Source: CAD feature listing. Evaluate the final solid. Frame: model axes, mm. A direction names the side the tool comes from. Give positions to 0.01 mm unless a question says otherwise; leave off trailing zeros.
from build123d import *

# Parameters (mm, degrees)
SKETCH1_R           = 2.4
BOSS_EXTRUDE1_DEPTH = 3.6


with BuildPart() as part:
    # Top → Base (revolve)
    with BuildSketch(Plane(origin=(0, 0, 0), x_dir=(1, 0, 0), z_dir=(0, 1, 0)), mode=Mode.PRIVATE) as base_sk:
        Polygon((-8.5, 32.9), (-8.5, 37.5), (-7, 37.5), (-7, 34.3), (-4.8, 34.3), (-4.8, 37.5), (-3.6, 37.5), (-3.6, 34.3), (3.6, 34.3), (3.6, 37.5), (4.8, 37.5), (4.8, 34.3), (7, 34.3), (7, 37.5), (8.5, 37.5), (8.5, 32.9), align=None)
    revolve(base_sk.sketch.rotate(Axis((0, 0, 0), (1, 0, 0)), 180), axis=Axis((0, 0, 0), (1, 0, 0)))

    # Sketch1 → Boss-Extrude1 (add, symmetric)
    with BuildSketch(Plane(origin=(0, 0, 0), x_dir=(0, 0, -1), z_dir=(1, 0, 0))):
        with BuildLine():
            Line((-2.132100415, 11.809070574), (-3.714992228, 32.689582939))
            ThreePointArc((-3.714992228, 32.689582939), (-4.659447617, 32.568382642), (-5.6, 32.419901295))
            Line((-5.6, 32.419901295), (-4, 11.313708499))
            ThreePointArc((-4, 11.313708499), (-5.797958971, 10.042359518), (-7.797958971, 9.120955865))
            Line((-7.797958971, 9.120955865), (-25.27645811, 21.059692909))
            ThreePointArc((-25.27645811, 21.059692909), (-25.875322919, 20.319391325), (-26.452513151, 19.562069114))
            Line((-26.452513151, 19.562069114), (-9.160904905, 7.75098841))
            ThreePointArc((-9.160904905, 7.75098841), (-10.392304845, 6), (-11.29300532, 4.058082164))
            Line((-11.29300532, 4.058082164), (-30.167505379, 13.127513825))
            ThreePointArc((-30.167505379, 13.127513825), (-30.534770537, 12.248991317), (-30.87645811, 11.360208386))
            Line((-30.87645811, 11.360208386), (-11.797958971, 2.192752634))
            ThreePointArc((-11.797958971, 2.192752634), (-11.595917942, 0), (-11.797958971, -2.192752634))
            Line((-11.797958971, -2.192752634), (-30.87645811, -11.360208386))
            ThreePointArc((-30.87645811, -11.360208386), (-30.534770537, -12.248991317), (-30.167505379, -13.127513825))
            Line((-30.167505379, -13.127513825), (-11.29300532, -4.058082164))
            ThreePointArc((-11.29300532, -4.058082164), (-10.392304845, -6), (-9.160904905, -7.75098841))
            Line((-9.160904905, -7.75098841), (-26.452513151, -19.562069114))
            ThreePointArc((-26.452513151, -19.562069114), (-25.875322919, -20.319391325), (-25.27645811, -21.059692909))
            Line((-25.27645811, -21.059692909), (-7.797958971, -9.120955865))
            ThreePointArc((-7.797958971, -9.120955865), (-5.797958971, -10.042359518), (-4, -11.313708499))
            Line((-4, -11.313708499), (-5.6, -32.419901295))
            ThreePointArc((-5.6, -32.419901295), (-4.659447617, -32.568382642), (-3.714992228, -32.689582939))
            Line((-3.714992228, -32.689582939), (-2.132100415, -11.809070574))
            ThreePointArc((-2.132100415, -11.809070574), (0, -12), (2.132100415, -11.809070574))
            Line((2.132100415, -11.809070574), (3.714992228, -32.689582939))
            ThreePointArc((3.714992228, -32.689582939), (4.659447617, -32.568382642), (5.6, -32.419901295))
            Line((5.6, -32.419901295), (4, -11.313708499))
            ThreePointArc((4, -11.313708499), (5.797958971, -10.042359518), (7.797958971, -9.120955865))
            Line((7.797958971, -9.120955865), (25.27645811, -21.059692909))
            ThreePointArc((25.27645811, -21.059692909), (25.875322919, -20.319391325), (26.452513151, -19.562069114))
            Line((26.452513151, -19.562069114), (9.160904905, -7.75098841))
            ThreePointArc((9.160904905, -7.75098841), (10.392304845, -6), (11.29300532, -4.058082164))
            Line((11.29300532, -4.058082164), (30.167505379, -13.127513825))
            ThreePointArc((30.167505379, -13.127513825), (30.534770537, -12.248991317), (30.87645811, -11.360208386))
            Line((30.87645811, -11.360208386), (11.797958971, -2.192752634))
            ThreePointArc((11.797958971, -2.192752634), (11.595917942, 0), (11.797958971, 2.192752634))
            Line((11.797958971, 2.192752634), (30.87645811, 11.360208386))
            ThreePointArc((30.87645811, 11.360208386), (30.534770537, 12.248991317), (30.167505379, 13.127513825))
            Line((30.167505379, 13.127513825), (11.29300532, 4.058082164))
            ThreePointArc((11.29300532, 4.058082164), (10.392304845, 6), (9.160904905, 7.75098841))
            Line((9.160904905, 7.75098841), (26.452513151, 19.562069114))
            ThreePointArc((26.452513151, 19.562069114), (25.875322919, 20.319391325), (25.27645811, 21.059692909))
            Line((25.27645811, 21.059692909), (7.797958971, 9.120955865))
            ThreePointArc((7.797958971, 9.120955865), (5.797958971, 10.042359518), (4, 11.313708499))
            Line((4, 11.313708499), (5.6, 32.419901295))
            ThreePointArc((5.6, 32.419901295), (4.659447617, 32.568382642), (3.714992228, 32.689582939))
            Line((3.714992228, 32.689582939), (2.132100415, 11.809070574))
            ThreePointArc((2.132100415, 11.809070574), (0, 12), (-2.132100415, 11.809070574))
        make_face()
        with Locations((0, 8)):
            Circle(SKETCH1_R, mode=Mode.SUBTRACT)
        Circle(SKETCH1_R, mode=Mode.SUBTRACT)
        with Locations((-6.92820323, 4)):
            Circle(SKETCH1_R, mode=Mode.SUBTRACT)
        with Locations((-6.92820323, -4)):
            Circle(SKETCH1_R, mode=Mode.SUBTRACT)
        with Locations((0, -8)):
            Circle(SKETCH1_R, mode=Mode.SUBTRACT)
        with Locations((6.92820323, -4)):
            Circle(SKETCH1_R, mode=Mode.SUBTRACT)
        with Locations((6.92820323, 4)):
            Circle(SKETCH1_R, mode=Mode.SUBTRACT)
    extrude(amount=BOSS_EXTRUDE1_DEPTH, both=True)


solid = part.part
1) First-contact query: pin 1 Ø1 at (x, z) = (-6, -17) entering from -Y; pin 2 Ø8 at (x, y) = (-3, -9) entering from -Z; pin 3 Ø1 at (y, z) = (-4.5, -14.5) entering from +X. Flat tips, straight axial feed; report the tip coordinate or a pass-through.
Checks:
pin 1: stops at y = -30.07
pin 2: stops at z = -37.16
pin 3: stops at x = 3.6
2) Reachability of faces 1 (the face through (3.6, 3, 2)), 2 (the face through (0.05, 8.656, -20.862)), 3 (the face through (-3.6, 30.4, 16.5)) from +Z, -Z, +X, -X, +Y, -Y: full face, straight path, thin tool, end or side. Return the list, or none.
Checks:
face 1: +X
face 2: +X, -X
face 3: none
3) Section query A-A on z = 0. State how many separate pieces and enclosed holes the cut face has, and give its area (3 significant figures).
Checks:
separate pieces: 6
enclosed holes: 0
area: 151 mm2
4) Pull-direction query (Z, two-part tool) for faces 4 (the face through (0.05, -15.007, -16.415)), 5 (the face through (7.76, 33.27, 17.3)), 6 (the face through (0.05, 22.103, 2.912)), 7 (the face through (3.6, 30.4, -16.5)); classes: +Z half, -Z half, draft (parallel to the pull), parting line (faces both ways), or undercut.
Checks:
face 4: undercut
face 5: parting line
face 6: undercut
face 7: draft
5) Ray query, L1, parallel to Z at x = 3.25, y = -3; L2, parallel to Y at x = 1.5, z = 8; L3, parallel to Y at x = 1.75, z = 6.5. Return the intervals inside material, ascending.
Checks:
L1: z = -34.17 to -32.76, -13.48 to -9.11, -4.75 to 4.75, 9.11 to 13.48, 32.76 to 34.17
L2: y = -33.35 to -31.91, -9.26 to -6.15, -1.85 to 1.85, 6.15 to 9.26, 31.91 to 33.35
L3: y = -33.68 to -32.25, -9.67 to -6.36, -1.64 to 1.64, 6.36 to 9.67, 32.25 to 33.68
